```python
from build123d import *

# Parameters (mm, degrees)
BOSS_EXTRUDE1_DEPTH = 1
SKETCH3_R           = 2.5
CUT_EXTRUDE2_DEPTH  = 2


with BuildPart() as part:
    # Sketch1 → Boss-Extrude1 (new, symmetric)
    with BuildSketch(Plane(origin=(0, 0, 0), x_dir=(1, 0, 0), z_dir=(0, 1, 0))):
        with BuildLine():
            Line((-15.654761905, 108.511904762), (-15.654761905, -41.488095238))
            ThreePointArc((-15.654761905, -41.488095238), (-8.154761905, -48.988095238), (-0.654761905, -41.488095238))
            Line((-0.654761905, -41.488095238), (-0.654761905, 108.511904762))
            ThreePointArc((-0.654761905, 108.511904762), (-8.154761905, 116.011904762), (-15.654761905, 108.511904762))
        make_face()
    extrude(amount=BOSS_EXTRUDE1_DEPTH, both=True)

    # Sketch3 → Cut-Extrude2 (cut)
    with BuildSketch(Plane(origin=(0, 1, 0), x_dir=(1, 0, 0), z_dir=(0, 1, 0))):
        with Locations(Location((-8.154761905, 108.511904762, 0), (0, 0, 270))):
            Circle(SKETCH3_R)
        with Locations(Location((-8.154761905, -41.488095238, 0), (0, 0, 270))):
            Circle(SKETCH3_R)
    extrude(amount=-CUT_EXTRUDE2_DEPTH, mode=Mode.SUBTRACT)


solid = part.part
```
Source: CAD feature listing. Evaluate the final solid. Frame: model axes, mm. Coordinates: 2 decimals unless noted, no trailing zeros. Loops run counter-clockwise (first coordinate to the right, second up) from the corner with the lowest first, then second, coordinate; pieces in that order, holes last. Notation, with made-up numbers: M 74.25,-18.5 L 115.25,-18.5 A22 cw 115.25,-8.5 Z; hole C 43.25,-11 d9. An arc over 180 degrees is marked long. Use a Markdown table: item, result. Add a question column.
Q1. Section query B-B, the plane x = -3.5. Return loops of the section in (y, z), and give its area (3 significant figures).
Q2. First-contact query: pin 1 (4 mm diameter, centred on x = -8.15, z = -108.51, fed in from -Y). Flat tip, straight axial feed; report the tip coordinate or a pass-through.
Q3. Section query C-C, the plane x = -14. Return loops of the section in (y, z).
Q4. Section query A-A, the plane y = -0.5. Return loops of the section in (x, z).
Q5. Material intervals for L1, parallel to Z at x = -8.25, y = 0.3; L2, parallel to Z at x = -7.5, y = 0; L3, parallel to X at y = 0, z = -107.5, sorted ascending.
Q6. Draft query along Z for faces 1 (the cylindrical face through (-8.32, 0.014, 48.986)), 2 (the cylindrical face through (-8.04, 0.01, -111.01)), 3 (the cylindrical face through (-7.99, 0.01, -116.01)). Return one class per face: pulls with the +Z half, pulls with the -Z half, needs draft (parallel to the pull), parting line crosses it, or undercut.
Result:
| question | item | result |
|---|---|---|
| 1 | outline | M -1,-114.39 L 1,-114.39 L 1,47.37 L -1,47.37 Z |
| 1 | area | 324 mm2 |
| 2 | pin 1 | passes through |
| 3 | outline | M -1,-113.21 L 1,-113.21 L 1,46.19 L -1,46.19 Z |
| 4 | outline | M -15.65,-108.51 A7.5 ccw -0.65,-108.51 L -0.65,41.49 A7.5 ccw -15.65,41.49 Z; hole C -8.15,-108.51 d5; hole C -8.15,41.49 d5 |
| 5 | L1 | z = -116.01 to -111.01, -106.01 to 38.99, 43.99 to 48.99 |
| 5 | L2 | z = -115.98 to -110.92, -106.1 to 39.08, 43.9 to 48.96 |
| 5 | L3 | x = -15.65 to -10.44, -5.87 to -0.65 |
| 6 | face 1 | pulls with the +Z half |
| 6 | face 2 | undercut |
| 6 | face 3 | pulls with the -Z half |
